Print and shaded views of the part. All mm, measured from the part's lowest x, y and z. A direction names the side the tool comes from. Round coordinates to 2 decimals unless told otherwise and drop trailing zeros. Write each loop counter-clockwise with the first axis right and the second up, starting at its lowest first coordinate (ties: lowest second). Pieces come first, ordered by that corner, then holes. Notation, with made-up numbers: (9, 22) -> (14, 22) arc R21 cw to (14, 43) -> close; hole circle Ø9 at (-8, -39). An arc over 180 degrees is marked (long way). Use CSV: the item, a comma, the result in double quotes. Start each with the question number.
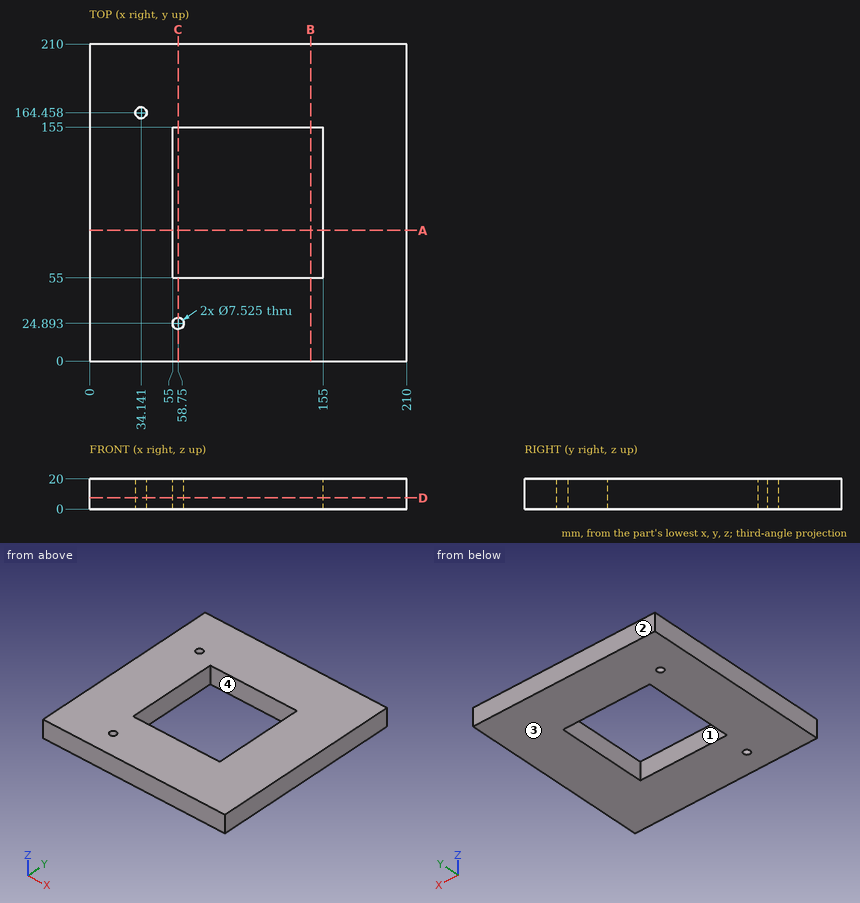
1. Band-saw the part on D-D (z = 7.5). Give the number of separate pieces and of enclosed holes in the cut face, then the cut area to 3 significant figures.
2. Drill centre lines: line 1 along Y through (x, z) = (58.75, 5.75) (1 decimal); line 2 along Y through (x, z) = (102, 14). Where is each one in solid material? Low to high. Write a range as [from, to].
3. Band-saw the part on A-A (y = 86.5). List the corners of the cut face in (x, z), then the cut area to 3 significant figures.
4. Which spindle directions (+Z, -Z, +X, -X, +Y, -Y) get a long thin tool onto all of the face, cutting with end or side? Do the marked faces 3 and 4. Say none if no direction does.
5. Pull direction X, two halves, no side cores. Call the marked faces 1 and 2: released by +X, released by -X, zero draft, split by the parting line, or undercut.
6. Band-saw the part on C-C (x = 58.75). List the corners of the cut face in (y, z) (1 decimal).
Answers below:
1,separate pieces,"1"
1,enclosed holes,"3"
1,area,"34,000 mm^2"
2,line 1,"y = [0, 21.1], [28.7, 55], [155, 210]"
2,line 2,"y = [0, 55], [155, 210]"
3,outline,"(0, 0) -> (55, 0) -> (55, 20) -> (0, 20) -> close; (155, 0) -> (210, 0) -> (210, 20) -> (155, 20) -> close"
3,area,"2,200 mm^2"
4,face 3,"-Z, +X, -X, +Y, -Y"
4,face 4,"+Z, -Z"
5,face 1,"undercut"
5,face 2,"zero draft"
6,outline,"(0, 0) -> (21.1, 0) -> (21.1, 20) -> (0, 20) -> close; (28.7, 0) -> (55, 0) -> (55, 20) -> (28.7, 20) -> close; (155, 0) -> (210, 0) -> (210, 20) -> (155, 20) -> close"
